from build123d import *

# Parameters (mm, degrees)
SKETCH1_R           = 11.136121628
BOSS_EXTRUDE1_DEPTH = 50.8
SKETCH2_W           = 22.261321628
SKETCH2_H           = 25.4
BOSS_EXTRUDE2_DEPTH = 3.834635566
SKETCH3_W           = 63.5
SKETCH3_H           = 2.530898103
BOSS_EXTRUDE3_DEPTH = 50.8
SKETCH4_W           = 4.132939296
SKETCH4_H           = 40.630898103
BOSS_EXTRUDE4_DEPTH = 50.8
SKETCH5_W           = 29.532939296
SKETCH5_H           = 4.001701266
BOSS_EXTRUDE5_DEPTH = 50.8
SKETCH6_W           = 22.261321628
SKETCH6_H           = 25.4
BOSS_EXTRUDE6_DEPTH = 3.834635566
FILLET2_R           = 5.08


with BuildPart() as part:
    # Sketch1 → Boss-Extrude1 (new body)
    with BuildSketch(Plane.YZ):
        with Locations(Location((0, 0, 0), (0, 0, 270))):
            Circle(SKETCH1_R)
    extrude(amount=BOSS_EXTRUDE1_DEPTH)

    # Sketch2 → Boss-Extrude2 (add)
    with BuildSketch(Plane(origin=(0, 0, 0), x_dir=(0, -1, 0), z_dir=(-1, 0, 0))):
        with Locations((-0.005460814, 12.7)):
            Rectangle(SKETCH2_W, SKETCH2_H)
    extrude(amount=-BOSS_EXTRUDE2_DEPTH)

    # Sketch3 → Boss-Extrude3 (add)
    with BuildSketch(Plane.YZ):
        with Locations((0, 26.665449052)):
            Rectangle(SKETCH3_W, SKETCH3_H)
    extrude(amount=BOSS_EXTRUDE3_DEPTH)

    # Sketch4 → Boss-Extrude4 (add)
    with BuildSketch(Plane.YZ):
        with Locations((-33.816469648, 45.715449052)):
            Rectangle(SKETCH4_W, SKETCH4_H)
        with Locations((33.816469648, 45.715449052)):
            Rectangle(SKETCH4_W, SKETCH4_H)
    extrude(amount=BOSS_EXTRUDE4_DEPTH)

    # Sketch5 → Boss-Extrude5 (add)
    with BuildSketch(Plane.YZ):
        with Locations((-21.116469648, 68.031748736)):
            Rectangle(SKETCH5_W, SKETCH5_H)
        with Locations((21.116469648, 68.031748736)):
            Rectangle(SKETCH5_W, SKETCH5_H)
    extrude(amount=BOSS_EXTRUDE5_DEPTH)

    # Sketch6 → Boss-Extrude6 (add)
    with BuildSketch(Plane.YZ.offset(50.8)):
        with Locations((0.005460814, 12.7)):
            Rectangle(SKETCH6_W, SKETCH6_H)
    extrude(amount=-BOSS_EXTRUDE6_DEPTH)

    # Fillet2
    fillet2_edges = [part.edges().sort_by_distance(p)[0] for p in [
        (1.917317783, 11.136121628, 25.4),
        (3.834635566, 0.005460814, 25.4),
        (1.917317783, -11.1252, 25.4),
        (46.965364434, 0.005460814, 25.4),
        (48.882682217, -11.1252, 25.4),
        (48.882682217, 11.136121628, 25.4),
    ]]
    fillet(fillet2_edges, radius=FILLET2_R)


solid = part.part
Work out the finished part from the listing and answer in its coordinate system (mm). A direction names the side the tool comes from. Coordinates: 2 decimals unless noted, no trailing zeros. Write each loop counter-clockwise with the first axis right and the second up, starting at its lowest first coordinate (ties: lowest second). Pieces come first, ordered by that corner, then holes. Notation, with made-up numbers: M 38.25,58 L 75.25,58 A8 cw 75.25,64 Z; hole C 78.25,74 d5. An arc over 180 degrees is marked long. Write item = value, one per line.
1. The part is cut by section B-B (z = 59). Determine the outline of the cut face in (x, y), then the cut area to 3 significant figures.
Solution:
outline = M 0,-35.88 L 50.8,-35.88 L 50.8,-31.75 L 0,-31.75 Z; M 0,31.75 L 50.8,31.75 L 50.8,35.88 L 0,35.88 Z
area = 420 mm2
2. The part is cut by section A-A (y = -22). Determine the outline of the cut face in (x, z).
Solution:
outline = M 0,25.4 L 50.8,25.4 L 50.8,27.93 L 0,27.93 Z; M 0,66.03 L 50.8,66.03 L 50.8,70.03 L 0,70.03 Z
3. Straight lines are drawn through the part: line 1 (Z direction, x = 31, y = 30.5); line 2 (Y direction, x = 6, z = 52); line 3 (Z direction, x = 33, y = 7). For each, find the intervals that lie inside material, in ascending order. Write a range as from..to.
Solution:
line_1 = 25.4..27.93, 66.03..70.03
line_2 = -35.88..-31.75, 31.75..35.88
line_3 = -8.66..8.66, 25.4..27.93, 66.03..70.03
4. Determine the mould class of faces 1 (the face through (50.8, 5, 27)), 2 (the face through (25, -1, 25.4)), 3 (the face through (0, -3, 24)) for opening direction X: released by +X, released by -X, zero draft, split by the parting line, or undercut.
Solution:
face_1 = released by +X
face_2 = undercut
face_3 = released by -X
5. Flat-ended cylindrical pins translate along their axes: pin 1 (12 mm diameter, centred on x = 14.5, z = 17.5, fed in from +Y) (3 decimals); pin 2 (4 mm diameter, centred on x = 49.5, z = 12, fed in from -Y); pin 3 (3 mm diameter, centred on x = 49.5, z = 6.5, fed in from +Y); pin 4 (4 mm diameter, centred on x = 9, z = 7.5, fed in from -Y). Find the tip coordinate at first contact, or state that the pin passes through.
Solution:
pin_1 = through
pin_2 = -11.13
pin_3 = 11.14
pin_4 = -9.68
6. The part is cut by section C-C (x = 27). Determine the outline of the cut face in (y, z), then the cut area to 3 significant figures.
Solution:
outline = M -35.88,25.4 L 35.88,25.4 L 35.88,70.03 L 6.35,70.03 L 6.35,66.03 L 31.75,66.03 L 31.75,27.93 L -31.75,27.93 L -31.75,66.03 L -6.35,66.03 L -6.35,70.03 L -35.88,70.03 Z; C 0,0 d22.27
area = 1,120 mm2
7. For faces 4 (the face through (49, -11.125, 10)), 5 (the face through (25, 6.35, 68)), 6 (the face through (5.28, -0.22, 23.87)), 7 (the face through (25, -31.75, 47)), determine the directions among +Z, -Z, +X, -X, +Y, -Y from which every point of the face is accessible in a straight line to the end or side of a thin tool.
Solution:
face_4 = -Z, +X, -X, -Y
face_5 = +Z, +X, -X
face_6 = +Y, -Y
face_7 = +X, -X
8. The part is cut by section D-D (y = 0). Determine the outline of the cut face in (x, z), then the cut area to 3 significant figures.
Solution:
outline = M 0,-11.14 L 50.8,-11.14 L 50.8,27.93 L 0,27.93 Z; hole M 3.83,11.14 L 46.97,11.14 L 46.97,20.32 A5.08 ccw 41.89,25.4 L 8.91,25.4 A5.08 ccw 3.83,20.32 Z
area = 1,380 mm2
